Geometry check sheet. Reference: the model listing, model coordinates, mm. Face numbers are marked on the shaded views. A direction names the side the tool comes from. Round coordinates to 2 decimals unless told otherwise and drop trailing zeros. Order: outer loops, then holes, each group sorted by start corner. A loop starts at its lowest first (then second) coordinate and runs counter-clockwise, first axis right, second up. Notation, with made-up numbers: M 56.5,50.5 L 109.5,50.5 A16 cw 109.5,78.5 Z; hole C -27.75,47 d5. An arc over 180 degrees is marked long. Answer as a JSON object with one key per item and string values. Group by question number.
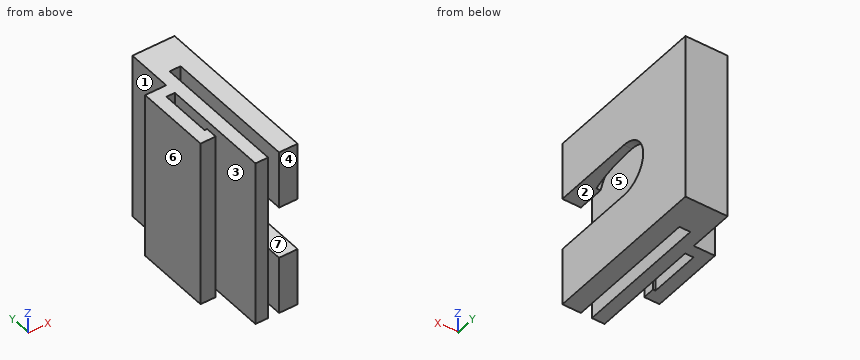
```python
from build123d import *
from build123d.topology import SkipClean

# Parameters (mm, degrees)
SKETCH1_W           = 4
SKETCH1_H           = 9
BOSS_EXTRUDE1_DEPTH = 20
SKETCH2_W           = 1
SKETCH2_H           = 6
CUT_EXTRUDE1_DEPTH  = 21.597329924
SKETCH4_W           = 20
SKETCH4_H           = 20
BOSS_EXTRUDE2_DEPTH = 1.5
SKETCH5_W           = 20
SKETCH5_H           = 20
BOSS_EXTRUDE3_DEPTH = 3.5
SKETCH7_W           = 1.8
SKETCH7_H           = 20
CUT_EXTRUDE5_DEPTH  = 16
CUT_EXTRUDE6_START  = -1.7
CUT_EXTRUDE6_DEPTH  = 1.7
BOSS_EXTRUDE4_START = 0.5
BOSS_EXTRUDE4_DEPTH = 0.5
SKETCH10_W          = 0.7
SKETCH10_H          = 1.5
CUT_EXTRUDE7_DEPTH  = 24.027157903
SKETCH11_W          = 1
SKETCH11_H          = 6.2
CUT_EXTRUDE8_DEPTH  = 24.027157903


with BuildPart() as part:
    # Sketch1 → Boss-Extrude1 (new body)
    with BuildSketch(Plane.XY):
        Rectangle(SKETCH1_W, SKETCH1_H)
    extrude(amount=BOSS_EXTRUDE1_DEPTH)

    # Sketch2 → Cut-Extrude1 (cut, through all)
    with BuildSketch(Plane(origin=(0, 0, 0), x_dir=(-1, 0, 0), z_dir=(0, 0, -1))):
        Rectangle(SKETCH2_W, SKETCH2_H)
    extrude(amount=-CUT_EXTRUDE1_DEPTH, mode=Mode.SUBTRACT)

    # Sketch4 → Boss-Extrude2 (add)
    with BuildSketch(Plane(origin=(2, 0, 0), x_dir=(0, 0, -1), z_dir=(1, 0, 0))):
        with Locations((-10, 0)):
            Rectangle(SKETCH4_W, SKETCH4_H)
    extrude(amount=-BOSS_EXTRUDE2_DEPTH)

    # Sketch5 → Boss-Extrude3 (add)
    with BuildSketch(Plane(origin=(2, 0, 0), x_dir=(0, 0, -1), z_dir=(1, 0, 0))):
        with Locations((-10, 0)):
            Rectangle(SKETCH5_W, SKETCH5_H)
    extrude(amount=BOSS_EXTRUDE3_DEPTH)

    # Sketch6 → Cut-Revolve2 (revolve, cut)
    with BuildSketch(Plane(origin=(0, 0, 10), x_dir=(-1, 0, 0), z_dir=(0, 0, -1)), mode=Mode.PRIVATE) as cut_revolve2_sk:
        with BuildLine():
            Line((-2, 7.5), (-2, 0))
            Line((-2, 0), (-4.700284, 0))
            ThreePointArc((-4.700284, 0), (-4.474408022, 3.776920415), (-3.8, 7.5))
            Line((-3.8, 7.5), (-2, 7.5))
        make_face()
    revolve(cut_revolve2_sk.sketch.rotate(Axis((88.99, 0, 10), (-1, 0, 0)), 90), axis=Axis((88.99, 0, 10), (-1, 0, 0)), mode=Mode.SUBTRACT)

    # Sketch7 → Cut-Extrude5 (cut)
    with BuildSketch(Plane.XZ.offset(10)):
        with Locations((2.9, 10)):
            Rectangle(SKETCH7_W, SKETCH7_H)
    extrude(amount=-CUT_EXTRUDE5_DEPTH, mode=Mode.SUBTRACT)

    # Sketch8 → Cut-Extrude6 (cut)
    with BuildSketch(Plane(origin=(5.5, 0, 0), x_dir=(0, 0, -1), z_dir=(1, 0, 0)).offset(CUT_EXTRUDE6_START)):
        with BuildLine():
            Line((-6.875, 0), (-6.875, -10))
            ThreePointArc((-6.875, -10), (-10, -13.125), (-13.125, -10))
            Line((-13.125, -10), (-13.125, 0))
            ThreePointArc((-13.125, 0), (-10, 3.125), (-6.875, 0))
        make_face()
    extrude(amount=CUT_EXTRUDE6_DEPTH, mode=Mode.SUBTRACT)

    # Sketch9 → Boss-Extrude4 (add)
    with SkipClean():  # the faces are left unmerged after this step: merging them gives an invalid solid
        with BuildSketch(Plane.ZY.offset(-3.8).offset(BOSS_EXTRUDE4_START)):
            with BuildLine():
                Line((13.125, -6.817945072), (13.125, -10))
                Line((13.125, -10), (20, -10))
                Line((20, -10), (20, 6))
                Line((20, 6), (14.5, 6))
                ThreePointArc((14.5, 6), (17.457216989, -0.799946739), (13.125, -6.817945072))
            make_face()
            with BuildLine():
                Line((0, -10), (6.875, -10))
                Line((6.875, -10), (6.875, -6.817945072))
                ThreePointArc((6.875, -6.817945072), (2.542783011, -0.799946739), (5.5, 6))
                Line((5.5, 6), (0, 6))
                Line((0, 6), (0, -10))
            make_face()
        extrude(amount=-BOSS_EXTRUDE4_DEPTH)

    # Sketch10 → Cut-Extrude7 (cut, through all)
    with SkipClean():  # the faces are left unmerged after this step: merging them gives an invalid solid
        with BuildSketch(Plane.XY.offset(20)):
            with Locations((0.15, -3.75)):
                Rectangle(SKETCH10_W, SKETCH10_H)
        extrude(amount=-CUT_EXTRUDE7_DEPTH, mode=Mode.SUBTRACT)

    # Sketch11 → Cut-Extrude8 (cut, through all)
    with SkipClean():  # the faces are left unmerged after this step: merging them gives an invalid solid
        with BuildSketch(Plane.XY.offset(20)):
            Rectangle(SKETCH11_W, SKETCH11_H)
        extrude(amount=-CUT_EXTRUDE8_DEPTH, mode=Mode.SUBTRACT)


solid = part.part
```
1) Sectioned sample at D-D (y = -2). Record the boundary of the cut face in (x, z) (3 decimals), then the cut area to 3 significant figures.
2) Sectioned sample at C-C (z = 16). Record the boundary of the cut face in (x, y).
3) Set-up check for the marked faces 1, 2, 3 and 4: record each of +Z, -Z, +X, -X, +Y, -Y from which the full face is reachable in a straight line by a thin tool's end or side.
4) Thickness scan on line 1 along X through (y, z) = (-7.5, 15.75); line 2 along X through (y, z) = (-0.5, 12); line 3 along X through (y, z) = (9.25, 9.5). Record the ranges inside material, lowest first. Write a range as [from, to].
5) Sectioned sample at B-B (y = 2). Record the boundary of the cut face in (x, z).
6) Go/stop test with flat-tipped pins: P1, Ø1.6, axis at y = 6.5, z = 15, coming from the -X side; P2, Ø1.4, axis at x = -1, z = 15, coming from the -Y side; P3, Ø0.8, axis at x = -0.5, z = 5.5, coming from the +Y side. Record where each tip stops, or that it passes through.
7) Release check for a two-part mould opening along X. For the marked faces 5, 6 and 7 record: +X half, -X half, draft (parallel to the pull), parting line (faces both ways), or undercut.
8) Sectioned sample at A-A (x = 5). Record the boundary of the cut face in (y, z) (3 decimals).
Final values:
{
 "1": {"outline": "M -2,0 L -0.5,0 L -0.5,20 L -2,20 Z; M 0.5,0 L 2,0 L 2,20 L 0.5,20 Z; M 3.3,0 L 5.5,0 L 5.5,6.875 L 4.482,6.875 A31.627 cw 3.8,2.772 L 3.3,2.772 Z; M 3.3,17.228 L 3.8,17.228 A31.627 cw 4.482,13.125 L 5.5,13.125 L 5.5,20 L 3.3,20 Z", "area": "83.0 mm^2"},
 "2": {"outline": "M -2,-4.5 L -0.2,-4.5 L -0.2,-3.1 L -0.5,-3.1 L -0.5,3.1 L 0.5,3.1 L 0.5,-10 L 2,-10 L 2,6 L 3.3,6 L 3.3,4.5 L 3.8,4.5 A31.12 cw 3.8,-4.5 L 3.3,-4.5 L 3.3,-10 L 5.5,-10 L 5.5,10 L 0.5,10 L 0.5,4.5 L -2,4.5 Z"},
 "3": {"face 1": "+Z, -Z, -X, +Y", "face 2": "+X, -Y", "face 3": "+Z, -Z, -Y", "face 4": "+Z, -Z, +X, -X, -Y"},
 "4": {"line 1": "x = [0.5, 2], [3.3, 5.5]", "line 2": "x = [-2, -0.5], [0.5, 2]", "line 3": "x = [0.5, 5.5]"},
 "5": {"outline": "M -2,0 L -0.5,0 L -0.5,20 L -2,20 Z; M 0.5,0 L 2,0 L 2,20 L 0.5,20 Z; M 3.3,0 L 5.5,0 L 5.5,7.6 L 4.55,7.6 A31.63 cw 3.8,2.77 L 3.3,2.77 Z; M 3.3,17.23 L 3.8,17.23 A31.63 cw 4.55,12.4 L 5.5,12.4 L 5.5,20 L 3.3,20 Z"},
 "6": {"P1": "stops at x = 0.5", "P2": "stops at y = -4.5", "P3": "stops at y = 4.5"},
 "7": {"face 5": "undercut", "face 6": "-X half", "face 7": "draft"},
 "8": {"outline": "M -10,0 L 10,0 L 10,20 L -10,20 L -10,13.125 L 0,13.125 A3.125 cw 0,6.875 L -10,6.875 Z"}
}
